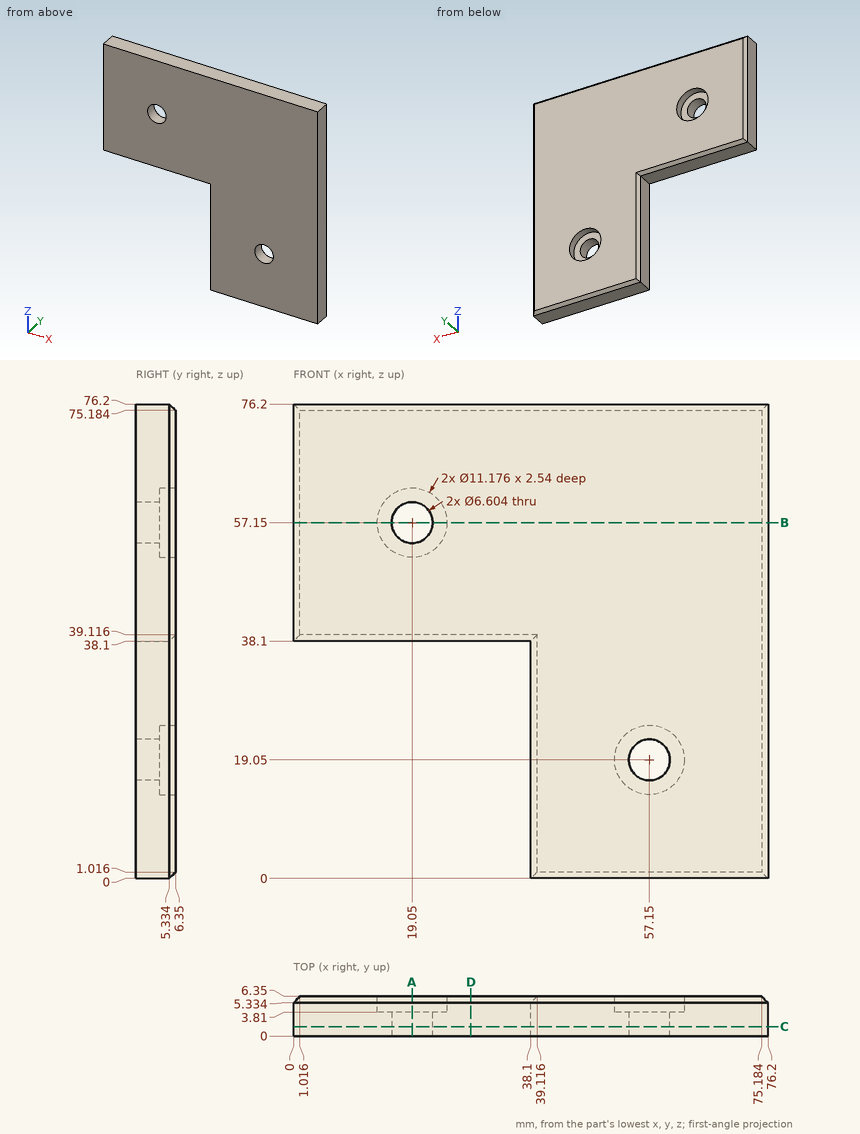
Verification items for this drawing (mm, ordinates from the low corner). Coordinates: 2 decimals unless noted, no trailing zeros. Write each loop counter-clockwise with the first axis right and the second up, starting at its lowest first coordinate (ties: lowest second). Pieces come first, ordered by that corner, then holes. Notation, with made-up numbers: M -13,17 L 16,17 A30 cw 16,56 Z; hole C 36,67 d3. An arc over 180 degrees is marked long. Use one line per item in the form item = value. Start each with the question number.
1) Section check C-C on y = 1.5. Enter the section's corners in (x, z).
2) Section check B-B on z = 57.15. Enter the section's corners in (x, y), and give its area (3 significant figures).
3) Section check D-D on x = 28.5. Enter the section's corners in (y, z).
4) Go/stop test with flat-tipped pins: pin 1 Ø1.6 at (x, y) = (12.5, 3.5) entering from -Z; pin 2 Ø3.5 at (x, z) = (56.5, 17.5) entering from +Y; pin 3 Ø2.5 at (y, z) = (3, 21.5) entering from -X. Record where each tip stops, or that it passes through.
5) Section check A-A on x = 19.05. Enter the section's corners in (y, z), and give its area (3 significant figures).
6) Thickness scan on probe 1 along Z at (x, y) = (57.15, 2.65); probe 2 along X at (y, z) = (1.2, 19.05); probe 3 along X at (y, z) = (4.7, 19.05). Record the ranges inside material, lowest first. Write a range as from..to.
Responses:
q1.outline = M 0,38.1 L 38.1,38.1 L 38.1,0 L 76.2,0 L 76.2,76.2 L 0,76.2 Z; hole C 19.05,57.15 d6.6; hole C 57.15,19.05 d6.6
q2.outline = M 0,0 L 15.75,0 L 15.75,3.81 L 13.46,3.81 L 13.46,6.35 L 1.02,6.35 L 0,5.33 Z; M 22.35,0 L 76.2,0 L 76.2,5.33 L 75.18,6.35 L 24.64,6.35 L 24.64,3.81 L 22.35,3.81 Z
q2.area = 429 mm2
q3.outline = M 0,38.1 L 5.33,38.1 L 6.35,39.12 L 6.35,75.18 L 5.33,76.2 L 0,76.2 Z
q4.pin_1 = 38.1
q4.pin_2 = 3.81
q4.pin_3 = 38.1
q5.outline = M 0,38.1 L 5.33,38.1 L 6.35,39.12 L 6.35,51.56 L 3.81,51.56 L 3.81,53.85 L 0,53.85 Z; M 0,60.45 L 3.81,60.45 L 3.81,62.74 L 6.35,62.74 L 6.35,75.18 L 5.33,76.2 L 0,76.2 Z
q5.area = 187 mm2
q6.probe_1 = 0..15.75, 22.35..76.2
q6.probe_2 = 38.1..53.85, 60.45..76.2
q6.probe_3 = 38.1..51.56, 62.74..76.2
